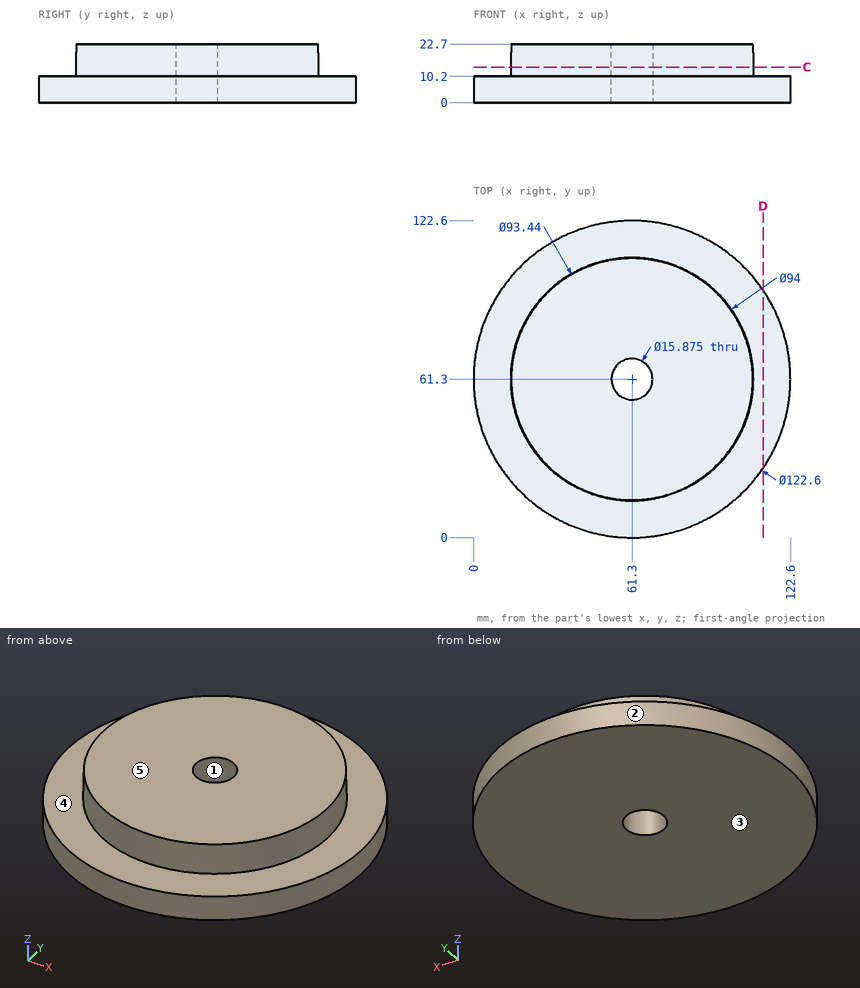
Verification items for this drawing (mm, ordinates from the low corner). A direction names the side the tool comes from. Give positions to 0.01 mm unless a question says otherwise; leave off trailing zeros. Loops run counter-clockwise (first coordinate to the right, second up) from the corner with the lowest first, then second, coordinate; pieces in that order, holes last. Notation, with made-up numbers: M -13.5,57.25 L -8.5,57.25 A23 ccw -8.5,78.25 Z; hole C 23,62.5 d6. An arc over 180 degrees is marked long. Answer as a JSON object with one key per item and string values. Group by question number.
Item 1: Sectioned sample at C-C on z = 13.75. Record the boundary of the cut face in (x, y) (1 decimal), plus the area to 3 significant figures.
Item 2: Access from +Z, -Z, +X, -X, +Y, -Y to the whole of each face (thin tool, end or side, straight path). Record for the marked faces 4 and 5.
Item 3: Gauge pin test, flat ends, axial feed: pin 1 (6 mm diameter, centred on y = 42.5, z = 17.5, fed in from +X); pin 2 (1 mm diameter, centred on x = 85, z = 9.5, fed in from -Y); pin 3 (6 mm diameter, centred on y = 19.5, z = 5, fed in from -X); pin 4 (14.5 mm diameter, centred on x = 61.3, y = 61.3, fed in from -Z). Record the tip position at first contact, or that the pin passes through.
Item 4: Material ranges on L1, parallel to Y at x = 61.3, z = 5.5; L2, parallel to X at y = 62, z = 17.5; L3, parallel to Z at x = 44.5, y = 13, recorded low to high.
Item 5: Sectioned sample at D-D on x = 112. Record the boundary of the cut face in (y, z).
Item 6: Mould release check, pull along X, two halves, no side actions. Record for the marked faces 1, 2 and 3: pulls with the +X half, pulls with the -X half, needs draft (parallel to the pull), parting line crosses it, or undercut.
Findings below:
{
 "1": {"outline": "C 61.3,61.3 d93.8; hole C 61.3,61.3 d15.9", "area": "6,720 mm2"},
 "2": {"face 4": "+Z", "face 5": "+Z, +X, -X, +Y, -Y"},
 "3": {"pin 1": "x = 105.39", "pin 2": "y = 4.56", "pin 3": "x = 13.84", "pin 4": "through"},
 "4": {"L1": "0 to 53.36, 69.24 to 122.6", "L2": "14.47 to 53.39, 69.21 to 108.13", "L3": "0 to 10.2"},
 "5": {"outline": "M 26.84,0 L 95.76,0 L 95.76,10.2 L 26.84,10.2 Z"},
 "6": {"face 1": "undercut", "face 2": "parting line crosses it", "face 3": "needs draft"}
}
